Autodesk Inventor part; units mm, degrees
ref_plane "YZ Plane" through (0, 0, 0) normal (1, 0, 0) x (0, 1, 0)
ref_plane "XZ Plane" through (0, 0, 0) normal (0, 1, 0) x (-1, 0, 0)
ref_plane "XY Plane" through (0, 0, 0) normal (0, 0, 1) x (1, 0, 0)
sketch "Sketch1" plane through (0, 0, 0) normal (0, 0, 1) x (1, 0, 0)
  line L0 (0, -8.5138) -> (0, 6.8862)
  line L1 (16, 3.5862) -> (16, -7.4138)
  line L2 (16, -7.4138) -> (20, -7.4138)
  line L3 (20, -7.4138) -> (20, -1.4138)
  line L4 (20, -1.4138) -> (25.5, -1.4138)
  line L5 (25.5, -1.4138) -> (25.5, 3.5862)
  line L6 (25.5, 3.5862) -> (16, 3.5862)
  dimension "d0" = 32
  dimension "d1" = 51
  dimension "d2" = 40
  dimension "d3" = 5
  dimension "d4" = 11
revolve "Revolution1" add sketch "Sketch1" angle 360 about axis through (0, -10, 0) along (0, 1, 0)
chamfer "Chamfer1" distance 5 angle 45 1 edges at (-16, 3.5862, 0)
properties part number "Seat" material "Bronze, Soft Tin"
The model under review builds one solid part; all positions refer to its coordinate system, in mm. A direction names the side the tool comes from. Round coordinates to 2 decimals unless told otherwise and drop trailing zeros. Write each loop counter-clockwise with the first axis right and the second up, starting at its lowest first coordinate (ties: lowest second). Pieces come first, ordered by that corner, then holes.
(1) Insertion check: pin 1 (3 mm diameter, centred on x = -11, y = -5, fed in from -Z); pin 2 (1.5 mm diameter, centred on y = -2.5, z = 4, fed in from -X); pin 3 (6 mm diameter, centred on y = -5, z = -16.5, fed in from -X). Each pin has a flat end and moves straight along its axis. Give the tip position at first contact, or say it passes through.
(2) We need section C-C on y = -2.5. Give the boundary of the cut face in (x, z), and give its area (3 significant figures).
(3) We need section D-D on y = 0.25. Give the boundary of the cut face in (x, z), and give its area (3 significant figures).
(4) Wall thickness on L1, parallel to X at y = -2.7, z = 0; L2, parallel to X at y = -1.75, z = 3: over which ranges is each line inside the solid? List them lowest first.
(5) Mouldability with a two-part tool opening along Z and no side actions: class faces 1 (the flat face through (-8.98, -7.414, -13.43)), 2 (the cylindrical face through (-4.336, -4.372, 19.524)), 3 (the conical face through (15.56, -1.1, -4.9)) as +Z half, -Z half, draft (parallel to the pull), parting line (faces both ways), or undercut.
(6) Machinability: for faces 4 (the flat face through (11, -1.414, 17)), 5 (the cylindrical face through (-5.5, 1.1, 24.9)), which of the approach directions +Z, -Z, +X, -X, +Y, -Y give a long, thin tool a straight path to every point of the face, cutting with its end or side? Answer none if there is none.
(7) We need section A-A on z = 0. Give the boundary of the cut face in (x, y).
(8) We need section B-B on x = 0. Give the boundary of the cut face in (y, z), and give its area (3 significant figures).
Findings below:
1. pin 1: stops at z = -17.6
1. pin 2: stops at x = -19.73
1. pin 3: stops at x = -14.76
2. outline: circle Ø40 at (0, 0); hole circle Ø32 at (0, 0)
2. area: 452 mm2
3. outline: circle Ø51 at (0, 0); hole circle Ø35.33 at (0, 0)
3. area: 1,060 mm2
4. L1: x = -20 to -16, 16 to 20
4. L2: x = -19.77 to -15.72, 15.72 to 19.77
5. face 1: draft
5. face 2: parting line
5. face 3: undercut
6. face 4: -Y
6. face 5: +Y, -Y
7. outline: (-25.5, -1.41) - (-20, -1.41) - (-20, -7.41) - (-16, -7.41) - (-16, -1.41) - (-21, 3.59) - (-25.5, 3.59) - close; (16, -7.41) - (20, -7.41) - (20, -1.41) - (25.5, -1.41) - (25.5, 3.59) - (21, 3.59) - (16, -1.41) - close
8. outline: (-7.41, -20) - (-1.41, -20) - (-1.41, -25.5) - (3.59, -25.5) - (3.59, -21) - (-1.41, -16) - (-7.41, -16) - close; (-7.41, 16) - (-1.41, 16) - (3.59, 21) - (3.59, 25.5) - (-1.41, 25.5) - (-1.41, 20) - (-7.41, 20) - close
8. area: 118 mm2
